Geometry: final body of the model. Coordinates: model frame, mm. A direction names the side the tool comes from. Coordinates: 2 decimals unless noted, no trailing zeros. Write each loop counter-clockwise with the first axis right and the second up, starting at its lowest first coordinate (ties: lowest second). Pieces come first, ordered by that corner, then holes.
from build123d import *

# Parameters (mm, degrees)
F1_R     = 2.65
F1_R_2   = 2.15
F1_R_3   = 8.1
F1_R_4   = 5
F1_R_5   = 1.65
F2_DEPTH = 5
F3_DEPTH = 3.9
F4_R     = 5


with BuildPart() as f2:
    # F1 (on Top) → F2 (new body)
    with BuildSketch(Plane.XY):
        with BuildLine():
            Line((-64.4537, 36.5492), (-64.6979, 35.0007))
            Line((-64.6979, 35.0007), (-64.6979, -34.9969))
            Line((-64.6979, -34.9969), (-64.4484, -36.5417))
            Line((-64.4484, -36.5417), (-63.7479, -37.9332))
            Line((-63.7479, -37.9332), (-62.6335, -39.0374))
            Line((-62.6335, -39.0374), (-61.2488, -39.7513))
            Line((-61.2488, -39.7513), (-59.7007, -39.9967))
            Line((-59.7007, -39.9967), (-4.979727, -39.999559))
            Line((-4.979727, -39.999559), (-1.17605, -50.300132))
            ThreePointArc((-1.17605, -50.300132), (6.0003, -55.300132), (13.17665, -50.300132))
            Line((13.17665, -50.300132), (16.979904, -40.000706))
            Line((16.979904, -40.000706), (20.6995, -40.0009))
            Line((20.6995, -40.0009), (21.4269, -39.9453))
            Line((21.4269, -39.9453), (22.1399, -39.7905))
            Line((22.1399, -39.7905), (22.8102, -39.5276))
            Line((22.8102, -39.5276), (51.9283, -25.9473))
            Line((51.9283, -25.9473), (52.4796, -25.5742))
            Line((52.4796, -25.5742), (52.8725, -25.0372))
            Line((52.8725, -25.0372), (53.0678, -24.3953))
            Line((53.0678, -24.3953), (53.6298, -22.2747))
            Line((53.6298, -22.2747), (54.7211, -20.3647))
            Line((54.7211, -20.3647), (56.2653, -18.7999))
            Line((56.2653, -18.7999), (58.1567, -17.6809))
            Line((58.1567, -17.6809), (60.2719, -17.0814))
            Line((60.2719, -17.0814), (62.4712, -17.0559))
            Line((62.4712, -17.0559), (63.308, -16.9719))
            Line((63.308, -16.9719), (64.0317, -16.5604))
            Line((64.0317, -16.5604), (64.5194, -15.8794))
            Line((64.5194, -15.8794), (64.6979, -15.0676))
            Line((64.6979, -15.0676), (64.6979, 15.0714))
            Line((64.6979, 15.0714), (64.5279, 15.8914))
            Line((64.5279, 15.8914), (64.0302, 16.5693))
            Line((64.0302, 16.5693), (63.3002, 16.9797))
            Line((63.3002, 16.9797), (62.4669, 17.0619))
            Line((62.4669, 17.0619), (60.2718, 17.0848))
            Line((60.2718, 17.0848), (58.1543, 17.681))
            Line((58.1543, 17.681), (56.2623, 18.8029))
            Line((56.2623, 18.8029), (54.7233, 20.3646))
            Line((54.7233, 20.3646), (53.6382, 22.281))
            Line((53.6382, 22.281), (53.0683, 24.401))
            Line((53.0683, 24.401), (52.8783, 25.0411))
            Line((52.8783, 25.0411), (52.4811, 25.5759))
            Line((52.4811, 25.5759), (51.9289, 25.9507))
            Line((51.9289, 25.9507), (22.812, 39.5287))
            Line((22.812, 39.5287), (22.1399, 39.7917))
            Line((22.1399, 39.7917), (21.4259, 39.9459))
            Line((21.4259, 39.9459), (20.6976, 40.0009))
            Line((20.6976, 40.0009), (16.98124, 40.000886))
            Line((16.98124, 40.000886), (13.17665, 50.303932))
            ThreePointArc((13.17665, 50.303932), (6.0003, 55.303932), (-1.17605, 50.303932))
            Line((-1.17605, 50.303932), (-4.980671, 40.000804))
            Line((-4.980671, 40.000804), (-59.6981, 40.0006))
            Line((-59.6981, 40.0006), (-61.245, 39.7556))
            Line((-61.245, 39.7556), (-62.6341, 39.0468))
            Line((-62.6341, 39.0468), (-63.7466, 37.9452))
            Line((-63.7466, 37.9452), (-64.4537, 36.5492))
        make_face()
        with Locations((-56.6982, -33.959099)):
            Circle(F1_R, mode=Mode.SUBTRACT)
        with Locations((-32.6989, -33.960634)):
            Circle(F1_R, mode=Mode.SUBTRACT)
        with Locations((-56.6957, -11.959936)):
            Circle(F1_R, mode=Mode.SUBTRACT)
        with Locations((-32.702, -11.964319)):
            Circle(F1_R, mode=Mode.SUBTRACT)
        with Locations((6.0003, -47.650132)):
            Circle(F1_R, mode=Mode.SUBTRACT)
        with Locations((0, -24.9981)):
            Circle(F1_R_2, mode=Mode.SUBTRACT)
        with Locations((32.6989, -13.962368)):
            Circle(F1_R, mode=Mode.SUBTRACT)
        with Locations((56.6944, -10.95745)):
            Circle(F1_R, mode=Mode.SUBTRACT)
        with Locations((-56.7023, 12.03785)):
            Circle(F1_R, mode=Mode.SUBTRACT)
        with Locations((-32.70075, 12.03915)):
            Circle(F1_R, mode=Mode.SUBTRACT)
        with Locations((-56.6982, 34.0357)):
            Circle(F1_R, mode=Mode.SUBTRACT)
        with Locations((-32.6997, 34.03845)):
            Circle(F1_R, mode=Mode.SUBTRACT)
        with Locations((0, 0.0019)):
            Circle(F1_R_3, mode=Mode.SUBTRACT)
        with Locations((20, 0.0019)):
            Circle(F1_R_4, mode=Mode.SUBTRACT)
        with Locations((0, 25.0019)):
            Circle(F1_R_2, mode=Mode.SUBTRACT)
        with Locations((56.703, 11.04075)):
            Circle(F1_R, mode=Mode.SUBTRACT)
        with Locations((32.698325, 14.036925)):
            Circle(F1_R, mode=Mode.SUBTRACT)
        with Locations((6.0003, 47.653932)):
            Circle(F1_R, mode=Mode.SUBTRACT)
        with Locations((0, 0.0019)):
            Circle(F1_R_3)
        with Locations((0, 0.0019)):
            Circle(F1_R_5, mode=Mode.SUBTRACT)
    extrude(amount=F2_DEPTH)

    # F1 (on Top) → F3 (cut)
    with BuildSketch(Plane.XY):
        with Locations((0, 0.0019)):
            Circle(F1_R_3)
        with Locations((0, 0.0019)):
            Circle(F1_R_5, mode=Mode.SUBTRACT)
    extrude(amount=F3_DEPTH, mode=Mode.SUBTRACT)

    # F4
    f4_edges = [f2.edges().sort_by_distance(p)[0] for p in [
        (-4.979727, -39.999559, 2.5),
        (16.979904, -40.000706, 2.5),
        (-4.980671, 40.000804, 2.5),
        (16.98124, 40.000886, 2.5),
    ]]
    fillet(f4_edges, radius=F4_R)


solid = f2.part
Item 1: Section B-B, the plane x = -11.5. Output: boundary loops of the cut face in (y, z), plus the area to 3 significant figures.
Derived:
outline: (-40, 0) - (40, 0) - (40, 5) - (-40, 5) - close
area: 400 mm2
Item 2: Material intervals for probe 1 along Y at (x, z) = (20, 4.4); probe 2 along X at (y, z) = (10, 3.75); probe 3 along X at (y, z) = (-34, 1.5), sorted ascending.
Derived:
probe 1: y = -40.02 to -5, 5 to 40.02
probe 2: x = -64.7 to -58.4, -55.01 to -34.39, -31.01 to 54.27, 59.14 to 64.7
probe 3: x = -64.7 to -59.35, -54.05 to -35.35, -30.05 to 34.66
Item 3: Pull-direction query (X, two-part tool) for faces 3 (the flat face through (-2.493, -46.735, 2.465)), 4 (the cylindrical face through (-57.043, 36.663, 2.465)), 5 (the flat face through (14.494, 46.737, 2.465)), 6 (the flat face through (-15, 1, 0)); classes: released by +X, released by -X, zero draft, split by the parting line, or undercut.
Derived:
face 3: released by -X
face 4: undercut
face 5: released by +X
face 6: zero draft
Item 4: Section A-A, the plane x = -32.5. Output: boundary loops of the cut face in (y, z).
Derived:
outline: (-40, 0) - (-36.6, 0) - (-36.6, 5) - (-40, 5) - close; (-31.32, 0) - (-14.61, 0) - (-14.61, 5) - (-31.32, 5) - close; (-9.32, 0) - (9.4, 0) - (9.4, 5) - (-9.32, 5) - close; (14.68, 0) - (31.4, 0) - (31.4, 5) - (14.68, 5) - close; (36.68, 0) - (40, 0) - (40, 5) - (36.68, 5) - close
Item 5: Set-up query: faces 1 (the cylindrical face through (17.6, -40.9, 2.5)), 2 (the flat face through (0, -2, 3.9)). Return all of +Z, -Z, +X, -X, +Y, -Y with unobstructed straight access to the full face (end or side cutting, diameter ignored); none if empty.
Derived:
face 1: +Z, -Z, +X, -Y
face 2: -Z
Item 6: Pin query (flat end, axial travel): pin 1 (2 mm diameter, centred on x = 50.5, z = 2, fed in from +Y); pin 2 (4 mm diameter, centred on x = 6, y = -47.65, fed in from -Z); pin 3 (1.5 mm diameter, centred on x = -41, z = 3, fed in from +Y); pin 4 (4 mm diameter, centred on x = 0, y = 0, fed in from -Z). Return the tip coordinate at first contact, or that it passes through.
Derived:
pin 1: stops at y = 27.08
pin 2: passes through
pin 3: stops at y = 40
pin 4: stops at z = 3.9
